from build123d import *

# Parameters (mm, degrees)
F1_DEPTH      = 50
F1_DEPTH_BACK = 50
F2_W          = 10
F2_H          = 45
F3_DEPTH      = 5
F4_R          = 6
F5_DEPTH      = 3
F6_R          = 4.99999


# Not quite as in the source:
# - a fillet or chamfer is up to 0.001 mm smaller than in the source, because OpenCascade refuses the exact size


with BuildPart() as f1:
    # F0 (on Top) → F1 (new body, two sides)
    with BuildSketch(Plane.XY) as f1_sk:
        Polygon((0, -12), (0, 0), (0, 20), (-10, 20), (-10, 0), (-34, 0), (-34, -12), align=None)
    extrude(amount=F1_DEPTH)
    extrude(f1_sk.sketch, amount=-F1_DEPTH_BACK)

    # F2 (on face) → F3 (join)
    with BuildSketch(Plane(origin=(0, 0, 0), x_dir=(-1, 0, 0), z_dir=(0, 1, 0))):
        with Locations((19, 5.5)):
            Rectangle(F2_W, F2_H)
    extrude(amount=F3_DEPTH)

    # F4 (on face) → F5 (cut)
    with BuildSketch(Plane(origin=(0, 0, 0), x_dir=(-1, 0, 0), z_dir=(0, 1, 0))):
        with Locations((22, 39)):
            Circle(F4_R)
        with Locations((22, -33.5)):
            Circle(F4_R)
    extrude(amount=-F5_DEPTH, mode=Mode.SUBTRACT)

    # F6 (radius 5 in the source; OpenCascade refuses exactly that, so slightly less here)
    f6_edges = [f1.edges().sort_by_distance(p)[0] for p in [
        (0, -12, 0),
        (0, 4, 50),
        (-17, -12, 50),
        (-17, -12, -50),
        (0, 4, -50),
        (-10, 20, 0),
        (0, 20, 0),
        (-34, 0, 0),
    ]]
    fillet(f6_edges, radius=F6_R)


solid = f1.part
Model file for the job. Use its own axes, mm. A direction names the side the tool comes from. Coordinates: 2 decimals unless noted, no trailing zeros. Loops run counter-clockwise (first coordinate to the right, second up) from the corner with the lowest first, then second, coordinate; pieces in that order, holes last. Notation, with made-up numbers: (-33, 55) -> (-16, 55) arc R13 cw to (-16, 67) -> close; hole circle Ø10 at (-22, -33). An arc over 180 degrees is marked (long way). Use one line per item in the form item = value. Start each with the question number.
(1) Tool access for faces 4 (the flat face through (-19, 2, 28)), 5 (the flat face through (-24, 2, 5)), 6 (the flat face through (-22, -3, -33)), 7 (the flat face through (-19, 2, -17)), 8 (the flat face through (-10, 8, 1)): list every direction of +Z, -Z, +X, -X, +Y, -Y with a clear straight run to the whole face (end or side of a thin tool).
(2) Cut at B-B on y = 7. Give the cut face in (x, z).
(3) Cut at A-A on x = -22. Give the cut face in (y, z), and give its area (3 significant figures).
(4) Flat gauge pins, fed straight in: pin 1 (9.5 mm diameter, centred on x = -24.5, z = 37.5, fed in from +Y); pin 2 (9.5 mm diameter, centred on x = -23.5, z = 5, fed in from +Y); pin 3 (16.5 mm diameter, centred on y = 10, z = 13.5, fed in from -X). Where does each tip first touch, or does it go through?
(5) Pull direction Z, two halves, no side cores. Call faces 1 (the cylindrical face through (-32, -1, -1)), 2 (the cylindrical face through (-19, -10, -49)), 3 (the cylindrical face through (-20.699, -1.479, 33.143)): pulls with the +Z half, pulls with the -Z half, needs draft (parallel to the pull), parting line crosses it, or undercut.
(6) Probe probe 1 along Z at (x, y) = (-22, -1.35); probe 2 along Y at (x, z) = (-17.5, -29); probe 3 along X at (y, z) = (10, -4). List the from-to ranges inside material, lowest first. Write a range as from..to.
Values:
q1.face_4 = +Z, -X, +Y
q1.face_5 = +Z, -Z, -X, +Y
q1.face_6 = +Y
q1.face_7 = -Z, -X, +Y
q1.face_8 = +Z, -Z, +Y
q2.outline = (-10, -50) -> (-5, -50) arc R5 ccw to (0, -45) -> (0, 45) arc R5 ccw to (-5, 50) -> (-10, 50) -> close
q3.outline = (-12, -45) arc R5 ccw to (-7, -50) -> (0, -50) -> (0, -39.5) -> (-3, -39.5) -> (-3, -27.5) -> (0, -27.5) -> (0, -17) -> (5, -17) -> (5, 28) -> (0, 28) -> (0, 33) -> (-3, 33) -> (-3, 45) -> (0, 45) -> (0, 50) -> (-7, 50) arc R5 ccw to (-12, 45) -> close
q3.area = 1,340 mm2
q4.pin_1 = 0
q4.pin_2 = 5
q4.pin_3 = -24
q5.face_1 = needs draft
q5.face_2 = pulls with the -Z half
q5.face_3 = undercut
q6.probe_1 = -50..-39.5, -27.5..33, 45..50
q6.probe_2 = -12..0
q6.probe_3 = -10..0
